Design review of the part built by this model. Coordinates are the model's own, in mm. Face numbers are marked on the shaded views. A direction names the side the tool comes from. Coordinates: 2 decimals unless noted, no trailing zeros. Loops run counter-clockwise (first coordinate to the right, second up) from the corner with the lowest first, then second, coordinate; pieces in that order, holes last. Notation, with made-up numbers: (-21, 24.25) -> (35, 24.25) arc R14 ccw to (35, 35.25) -> close; hole circle Ø11 at (-13, 79). An arc over 180 degrees is marked (long way). Use a Markdown table: item, result. Add a question column.
Q1. For probe 1 along Z at (x, y) = (-3, -21.5); probe 2 along Z at (x, y) = (17, -14.5); probe 3 along X at (y, z) = (-11, -139.5), list the stretches that pass through material, from the lowest coordinate up.
Q2. Clearance check with flat-ended pins moving along their axes: pin 1 Ø5 at (x, y) = (28, -3) entering from +Z; pin 2 Ø11 at (y, z) = (-17.5, -32) entering from -X; pin 3 Ø6 at (y, z) = (-19.5, -23.5) entering from +X. State where each tip first meets the part, or that it passes through.
Q3. For the marked faces 1, 2, 3, 4 and 5, list the 3-axis set-ups (+Z, -Z, +X, -X, +Y, -Y) from which the entire face can be reached by the end or side of a thin tool; tool diameter is ignored.
Q4. Take a section at D-D on z = -131.5. Write out the cut boundary in (x, y), plus the area to 3 significant figures.
Q5. Take a section at A-A on y = -19. Write out the cut boundary in (x, z), plus the area to 3 significant figures.
Q6. Draft analysis for pull direction X (two halves, no side actions). For the marked faces 6, 7 and 8, state which applies: pulls with the +X half, pulls with the -X half, needs draft (parallel to the pull), parting line crosses it, or undercut.
Q7. Take a section at C-C on x = 0. Write out the cut boundary in (y, z).
Q8. Take a section at B-B on z = -109.5. Write out the cut boundary in (x, y), plus the area to 3 significant figures.
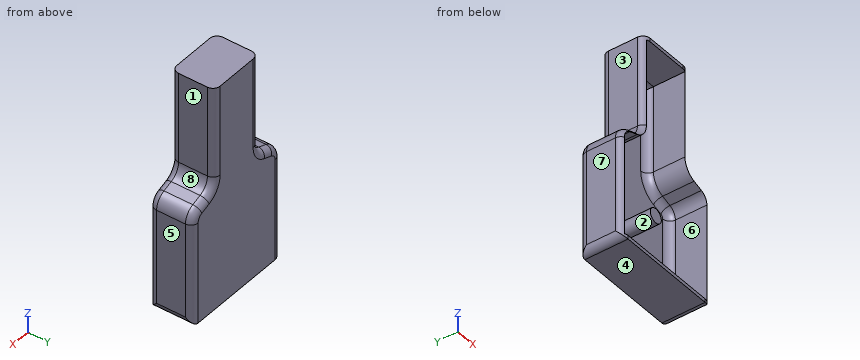
from build123d import *

# Parameters (mm, degrees)
F1_DEPTH     = 30
F2_T         = -2.5
F3_T1_DEPTH  = 55
F3_T3_DEPTH  = 83.3823547945
F3_T5_DEPTH  = 7.0343109423
F3_T7_DEPTH  = 75.4166657368
F3_T9_DEPTH  = 7.0343109423
F3_T12_ANGLE = 70.6224339747
F3_T14_ANGLE = 70.6224339747
F3_T16_ANGLE = 70.6224339747
F3_T18_ANGLE = 70.6224339747
F3_T20_ANGLE = 70.6224339747
F3_T22_ANGLE = 70.6224339747
F3_T24_ANGLE = 70.6224339747
F3_T26_ANGLE = 70.6224339747
F5_R         = 5
F6_DEPTH     = 20
F7_R         = 5


# Not quite as in the source:
# - a fillet or chamfer that OpenCascade refuses, or shapes differently, is made with other operations: its cross-section is extruded or revolved along the edge and cut away or added


with BuildPart() as f1:
    # F0 (on Front) → F1 (new body)
    with BuildSketch(Plane.XZ):
        with BuildLine():
            Line((20, 0), (0, 0))
            Line((0, 0), (-20, 0))
            Line((-20, 0), (-20, -62.9166657368))
            ThreePointArc((-20, -62.9166657368), (-21.8397555469, -68.6968396499), (-26.6820820931, -72.3501921592))
            Line((-26.6820820931, -72.3501921592), (-33.3179179069, -74.6841187831))
            ThreePointArc((-33.3179179069, -74.6841187831), (-38.1602444531, -78.3374712924), (-40, -84.1176452055))
            Line((-40, -84.1176452055), (-40, -155))
            Line((-40, -155), (0, -155))
            Line((0, -155), (40, -155))
            Line((40, -155), (40, -84.1176452055))
            ThreePointArc((40, -84.1176452055), (38.1602444531, -78.3374712924), (33.3179179069, -74.6841187831))
            Line((33.3179179069, -74.6841187831), (26.6820820931, -72.3501921592))
            ThreePointArc((26.6820820931, -72.3501921592), (21.8397555469, -68.6968396499), (20, -62.9166657368))
            Line((20, -62.9166657368), (20, 0))
        make_face()
    extrude(amount=F1_DEPTH)

    # F2
    f2_openings = [f1.faces().sort_by_distance(p)[0] for p in [
        (0, -30, -90.139239),
    ]]
    offset(amount=F2_T, openings=f2_openings)

    # F3: fillet of radius 5 on 8 edges, made by hand

    # F3_s2 → F3_t1 (cut)
    with BuildSketch(Plane.XZ.offset(-12.5)):
        with BuildLine():
            ThreePointArc((-35, -155), (-38.5355339059, -153.5355339059), (-40, -150))
            Line((-40, -150), (-40, -155))
            Line((-40, -155), (-35, -155))
        make_face()
        with BuildLine():
            ThreePointArc((40, -150), (38.5355339059, -153.5355339059), (35, -155))
            Line((35, -155), (40, -155))
            Line((40, -155), (40, -150))
        make_face()
    extrude(amount=F3_T1_DEPTH, mode=Mode.SUBTRACT)

    # F3_s4 → F3_t3 (cut)
    with BuildSketch(Plane.XY.offset(-167.5)):
        with BuildLine():
            ThreePointArc((-35, 0), (-38.5355339059, -1.4644660941), (-40, -5))
            Line((-40, -5), (-40, 0))
            Line((-40, 0), (-35, 0))
        make_face()
        with BuildLine():
            ThreePointArc((-40, -25), (-38.5355339059, -28.5355339059), (-35, -30))
            Line((-35, -30), (-40, -30))
            Line((-40, -30), (-40, -25))
        make_face()
        with BuildLine():
            ThreePointArc((35, 0), (38.5355339059, -1.4644660941), (40, -5))
            Line((40, -5), (40, 0))
            Line((40, 0), (35, 0))
        make_face()
        with BuildLine():
            ThreePointArc((40, -25), (38.5355339059, -28.5355339059), (35, -30))
            Line((35, -30), (40, -30))
            Line((40, -30), (40, -25))
        make_face()
    extrude(amount=F3_T3_DEPTH, mode=Mode.SUBTRACT)

    # F3_s6 → F3_t5 (cut)
    with BuildSketch(Plane(origin=(53.0259684291, 0, -18.6500574974), x_dir=(0, 1, 0), z_dir=(-0.9433526422, 0, 0.3317917907))):
        with BuildLine():
            ThreePointArc((-25, 59.3988491433), (-28.5355339059, 60.8633152374), (-30, 64.3988491433))
            Line((-30, 64.3988491433), (-30, 59.3988491433))
            Line((-30, 59.3988491433), (-25, 59.3988491433))
        make_face()
        with BuildLine():
            ThreePointArc((0, 64.3988491433), (-1.4644660941, 60.8633152374), (-5, 59.3988491433))
            Line((-5, 59.3988491433), (0, 59.3988491433))
            Line((0, 59.3988491433), (0, 64.3988491433))
        make_face()
    extrude(amount=F3_T5_DEPTH, mode=Mode.SUBTRACT)

    # F3_s8 → F3_t7 (cut)
    with BuildSketch(Plane.XY.offset(-62.9166657368)):
        with BuildLine():
            ThreePointArc((20, -25), (18.5355339059, -28.5355339059), (15, -30))
            Line((15, -30), (20, -30))
            Line((20, -30), (20, -25))
        make_face()
        with BuildLine():
            ThreePointArc((15, 0), (18.5355339059, -1.4644660941), (20, -5))
            Line((20, -5), (20, 0))
            Line((20, 0), (15, 0))
        make_face()
        with BuildLine():
            ThreePointArc((-20, -25), (-18.5355339059, -28.5355339059), (-15, -30))
            Line((-15, -30), (-20, -30))
            Line((-20, -30), (-20, -25))
        make_face()
        with BuildLine():
            ThreePointArc((-15, 0), (-18.5355339059, -1.4644660941), (-20, -5))
            Line((-20, -5), (-20, 0))
            Line((-20, 0), (-15, 0))
        make_face()
    extrude(amount=F3_T7_DEPTH, mode=Mode.SUBTRACT)

    # F3_s10 → F3_t9 (cut)
    with BuildSketch(Plane(origin=(-46.3901326153, 0, -16.3161308736), x_dir=(0, 1, 0), z_dir=(-0.9433526422, 0, -0.3317917907))):
        with BuildLine():
            ThreePointArc((-25, 59.3988491433), (-28.5355339059, 60.8633152374), (-30, 64.3988491433))
            Line((-30, 64.3988491433), (-30, 59.3988491433))
            Line((-30, 59.3988491433), (-25, 59.3988491433))
        make_face()
        with BuildLine():
            ThreePointArc((0, 64.3988491433), (-1.4644660941, 60.8633152374), (-5, 59.3988491433))
            Line((-5, 59.3988491433), (0, 59.3988491433))
            Line((0, 59.3988491433), (0, 64.3988491433))
        make_face()
    extrude(amount=F3_T9_DEPTH, mode=Mode.SUBTRACT)

    # F3_s11 → F3_t12 (revolve, cut)
    with BuildSketch(Plane.XY.offset(-84.1176452055)):
        with BuildLine():
            ThreePointArc((40, -25), (38.5355339059, -28.5355339059), (35, -30))
            Line((35, -30), (40, -30))
            Line((40, -30), (40, -25))
        make_face()
    revolve(axis=Axis((30, -30, -84.1176452055), (0, -1, 0)), revolution_arc=F3_T12_ANGLE, mode=Mode.SUBTRACT)

    # F3_s13 → F3_t14 (revolve, cut)
    with BuildSketch(Plane(origin=(46.3901326153, 0, -16.3161308736), x_dir=(0, 1, 0), z_dir=(0.9433526422, 0, -0.3317917907))):
        with BuildLine():
            ThreePointArc((-25, -59.3988491433), (-28.5355339059, -60.8633152374), (-30, -64.3988491433))
            Line((-30, -64.3988491433), (-30, -59.3988491433))
            Line((-30, -59.3988491433), (-25, -59.3988491433))
        make_face()
    revolve(axis=Axis((30, -30, -62.9166657368), (0, 1, 0)), revolution_arc=F3_T14_ANGLE, mode=Mode.SUBTRACT)

    # F3_s15 → F3_t16 (revolve, cut)
    with BuildSketch(Plane.XY.offset(-84.1176452055)):
        with BuildLine():
            ThreePointArc((35, 0), (38.5355339059, -1.4644660941), (40, -5))
            Line((40, -5), (40, 0))
            Line((40, 0), (35, 0))
        make_face()
    revolve(axis=Axis((30, 0, -84.1176452055), (0, -1, 0)), revolution_arc=F3_T16_ANGLE, mode=Mode.SUBTRACT)

    # F3_s17 → F3_t18 (revolve, cut)
    with BuildSketch(Plane(origin=(46.3901326153, 0, -16.3161308736), x_dir=(0, 1, 0), z_dir=(0.9433526422, 0, -0.3317917907))):
        with BuildLine():
            ThreePointArc((-5, -59.3988491433), (-1.4644660941, -60.8633152374), (0, -64.3988491433))
            Line((0, -64.3988491433), (0, -59.3988491433))
            Line((0, -59.3988491433), (-5, -59.3988491433))
        make_face()
    revolve(axis=Axis((30, 0, -62.9166657368), (0, 1, 0)), revolution_arc=F3_T18_ANGLE, mode=Mode.SUBTRACT)

    # F3_s19 → F3_t20 (revolve, cut)
    with BuildSketch(Plane(origin=(-53.0259684291, 0, -18.6500574974), x_dir=(0, 1, 0), z_dir=(0.9433526422, 0, 0.3317917907))):
        with BuildLine():
            ThreePointArc((-25, -59.3988491433), (-28.5355339059, -60.8633152374), (-30, -64.3988491433))
            Line((-30, -64.3988491433), (-30, -59.3988491433))
            Line((-30, -59.3988491433), (-25, -59.3988491433))
        make_face()
    revolve(axis=Axis((-30, -30, -84.1176452055), (0, -1, 0)), revolution_arc=F3_T20_ANGLE, mode=Mode.SUBTRACT)

    # F3_s21 → F3_t22 (revolve, cut)
    with BuildSketch(Plane.XY.offset(-62.9166657368)):
        with BuildLine():
            ThreePointArc((-20, -25), (-18.5355339059, -28.5355339059), (-15, -30))
            Line((-15, -30), (-20, -30))
            Line((-20, -30), (-20, -25))
        make_face()
    revolve(axis=Axis((-30, -30, -62.9166657368), (0, 1, 0)), revolution_arc=F3_T22_ANGLE, mode=Mode.SUBTRACT)

    # F3_s23 → F3_t24 (revolve, cut)
    with BuildSketch(Plane(origin=(-53.0259684291, 0, -18.6500574974), x_dir=(0, 1, 0), z_dir=(0.9433526422, 0, 0.3317917907))):
        with BuildLine():
            ThreePointArc((0, -64.3988491433), (-1.4644660941, -60.8633152374), (-5, -59.3988491433))
            Line((-5, -59.3988491433), (0, -59.3988491433))
            Line((0, -59.3988491433), (0, -64.3988491433))
        make_face()
    revolve(axis=Axis((-30, 0, -84.1176452055), (0, -1, 0)), revolution_arc=F3_T24_ANGLE, mode=Mode.SUBTRACT)

    # F3_s25 → F3_t26 (revolve, cut)
    with BuildSketch(Plane.XY.offset(-62.9166657368)):
        with BuildLine():
            ThreePointArc((-15, 0), (-18.5355339059, -1.4644660941), (-20, -5))
            Line((-20, -5), (-20, 0))
            Line((-20, 0), (-15, 0))
        make_face()
    revolve(axis=Axis((-30, 0, -62.9166657368), (0, 1, 0)), revolution_arc=F3_T26_ANGLE, mode=Mode.SUBTRACT)

    # F5 (on offset) → F6 (join)
    with BuildSketch(Plane.XZ.offset(22.5)):
        with Locations((0, -112.5)):
            Circle(F5_R)
    extrude(amount=-F6_DEPTH)

    # F7
    f7_edges = [f1.edges().sort_by_distance(p)[0] for p in [
        (-37.5, -2.5, -118.308823),
        (0, -2.5, -152.5),
        (0, -2.5, -2.5),
        (17.5, -2.5, -32.708333),
    ]]
    fillet(f7_edges, radius=F7_R)


solid = f1.part
Answer list:
| question | item | result |
|---|---|---|
| 1 | probe 1 | -155 to -152.5, -116.5 to -108.5, -2.5 to 0 |
| 1 | probe 2 | -155 to -152.5, -2.5 to 0 |
| 1 | probe 3 | -40 to -37.5, 37.5 to 40 |
| 2 | pin 1 | z = -72.06 |
| 2 | pin 2 | x = -20 |
| 2 | pin 3 | x = 20 |
| 3 | face 1 | +Z, +X, +Y, -Y |
| 3 | face 2 | -Y |
| 3 | face 3 | +Z, -X, +Y, -Y |
| 3 | face 4 | -Z, +X, -X, +Y, -Y |
| 3 | face 5 | +Z, -Z, +X, +Y, -Y |
| 4 | outline | (-40, -25) arc R5 ccw to (-37.5, -29.33) -> (-37.5, -7.5) arc R5 cw to (-32.5, -2.5) -> (32.5, -2.5) arc R5 cw to (37.5, -7.5) -> (37.5, -29.33) arc R5 ccw to (40, -25) -> (40, -5) arc R5 ccw to (35, 0) -> (-35, 0) arc R5 ccw to (-40, -5) -> close |
| 4 | area | 328 mm² |
| 5 | outline | (-40, -150) arc R5 ccw to (-35, -155) -> (35, -155) arc R5 ccw to (40, -150) -> (40, -84.12) arc R10 ccw to (33.32, -74.68) -> (26.68, -72.35) arc R10 cw to (20, -62.92) -> (20, 0) -> (-20, 0) -> (-20, -62.92) arc R10 cw to (-26.68, -72.35) -> (-33.32, -74.68) arc R10 ccw to (-40, -84.12) -> close; circle Ø10 at (0, -112.5); hole (-37.5, -152.5) -> (37.5, -152.5) -> (37.5, -84.12) arc R7.5 ccw to (32.49, -77.04) -> (25.85, -74.71) arc R12.5 cw to (17.5, -62.92) -> (17.5, -2.5) -> (-17.5, -2.5) -> (-17.5, -62.92) arc R12.5 cw to (-25.85, -74.71) -> (-32.49, -77.04) arc R7.5 ccw to (-37.5, -84.12) -> close |
| 5 | area | 1,170 mm² |
| 6 | face 6 | undercut |
| 6 | face 7 | pulls with the -X half |
| 6 | face 8 | pulls with the +X half |
| 7 | outline | (-30, -155) -> (0, -155) -> (0, 0) -> (-30, 0) -> (-30, -2.5) -> (-7.5, -2.5) arc R5 cw to (-2.5, -7.5) -> (-2.5, -107.5) -> (-22.5, -107.5) -> (-22.5, -117.5) -> (-2.5, -117.5) -> (-2.5, -147.5) arc R5 cw to (-7.5, -152.5) -> (-30, -152.5) -> close |
| 8 | outline | (-40, -25) arc R5 ccw to (-37.5, -29.33) -> (-37.5, -7.5) arc R5 cw to (-32.5, -2.5) -> (-4, -2.5) -> (-4, -22.5) -> (4, -22.5) -> (4, -2.5) -> (32.5, -2.5) arc R5 cw to (37.5, -7.5) -> (37.5, -29.33) arc R5 ccw to (40, -25) -> (40, -5) arc R5 ccw to (35, 0) -> (-35, 0) arc R5 ccw to (-40, -5) -> close |
| 8 | area | 488 mm² |
